Input: part model. Units: mm. Frame: model coordinates. A direction names the side the tool comes from. Round coordinates to 2 decimals unless told otherwise and drop trailing zeros. Order: outer loops, then holes, each group sorted by start corner. A loop starts at its lowest first (then second) coordinate and runs counter-clockwise, first axis right, second up.
Item 1: Cut plane D-D on y = 5.5. Give the number of separate pieces and of enclosed holes in the cut face, then the cut area to 3 significant figures.
Item 2: Cut plane C-C on x = 19. Output: boundary loops of the cut face in (y, z), then the cut area to 3 significant figures.
Item 3: Line query: L1, parallel to X at y = 1.5, z = 34; L2, parallel to Z at x = 0, y = 4.6; L3, parallel to X at y = 6.1, z = 0. Output: solid intervals per line, ascending.
Item 4: Cut plane A-A on z = 0. Output: boundary loops of the cut face in (x, y).
Item 5: First-contact query: pin 1 (4 mm diameter, centred on y = 3.5, z = 2, fed in from -X); pin 2 (0.8 mm diameter, centred on y = 6.5, z = 3, fed in from +X); pin 3 (2 mm diameter, centred on x = -37.5, y = 3.5, fed in from -Z). Flat tips, straight axial feed; report the tip coordinate or a pass-through.
Item 6: Reachability of faces 1 (the flat face through (25, 6, -4.5)), 2 (the flat face through (-16.61, 3.7, -23.68)), 3 (the flat face through (31, 6, 3.651)) from +Z, -Z, +X, -X, +Y, -Y: full face, straight path, thin tool, end or side. Return the list, or none.
Item 7: Cut plane B-B on x = 0. Output: boundary loops of the cut face in (y, z), then the cut area to 3 significant figures.
Item 8: Mould query, pull axis X, two halves, no side actions, for faces 4 (the flat face through (41.449, 4, 31)), 5 (the cylindrical face through (38.9, 3.8, 31.54)), 6 (the flat face through (36.559, 3.698, 36.648)), 7 (the flat face through (0, 0, -12)). Classes: released by +X, released by -X, zero draft, split by the parting line, or undercut.
```python
from build123d import *

# Parameters (mm, degrees)
SKETCH1_R           = 2.5
BOSS_EXTRUDE1_DEPTH = 7.5
FILLET3_R           = 1.5
SKETCH3_W           = 25.4
SKETCH3_H           = 9
CUT_EXTRUDE1_DEPTH  = 2
SKETCH2_W           = 24.748800006
SKETCH2_H           = 9
SKETCH2_W_2         = 9
SKETCH2_H_2         = 1.651
BOSS_EXTRUDE3_DEPTH = 3
SKETCH4_W           = 24.748800006
SKETCH4_H           = 9
BOSS_EXTRUDE4_DEPTH = 1


with BuildPart() as part:
    # Sketch1 → Boss-Extrude1 (new body)
    with BuildSketch(Plane(origin=(0, 0, 0), x_dir=(1, 0, 0), z_dir=(0, 1, 0))):
        Polygon((-41.448800006, 34.091704203), (-34.091704203, 41.448800006), (-27.292890359, 41.448800006), (-27.292890359, 34.363958171), (-5.628932188, 12.7), (5.628932188, 12.7), (27.292890359, 34.363958171), (27.292890359, 41.448800006), (34.091704203, 41.448800006), (41.448800006, 34.091704203), (41.448800006, 27.292890359), (34.363958171, 27.292890359), (12.7, 5.628932188), (12.7, -5.628932188), (34.363958171, -27.292890359), (41.448800006, -27.292890359), (41.448800006, -34.091704203), (34.091704203, -41.448800006), (27.292890359, -41.448800006), (27.292890359, -34.363958171), (5.628932188, -12.7), (-5.628932188, -12.7), (-27.292890359, -34.363958171), (-27.292890359, -41.448800006), (-34.091704203, -41.448800006), (-41.448800006, -34.091704203), (-41.448800006, -27.292890359), (-34.363958171, -27.292890359), (-12.7, -5.628932188), (-12.7, 5.628932188), (-34.363958171, 27.292890359), (-41.448800006, 27.292890359), align=None)
        with Locations(Location((0, 0, 0), (0, 0, 270))):
            Circle(SKETCH1_R, mode=Mode.SUBTRACT)
        Polygon((-39.798800006, 33.408251825), (-33.408251825, 39.798800006), (-29.292890359, 39.798800006), (-39.798800006, 29.292890359), align=None, mode=Mode.SUBTRACT)
        Polygon((-33.408251825, -39.798800006), (-29.292890359, -39.798800006), (-39.798800006, -29.292890359), (-39.798800006, -33.408251825), align=None, mode=Mode.SUBTRACT)
        Polygon((39.798800006, -33.408251825), (39.798800006, -29.292890359), (29.292890359, -39.798800006), (33.408251825, -39.798800006), align=None, mode=Mode.SUBTRACT)
        Polygon((33.408251825, 39.798800006), (39.798800006, 33.408251825), (39.798800006, 29.292890359), (29.292890359, 39.798800006), align=None, mode=Mode.SUBTRACT)
    extrude(amount=BOSS_EXTRUDE1_DEPTH)

    # Fillet3
    fillet3_edges = [part.edges().sort_by_distance(p)[0] for p in [
        (39.798800006, 3.75, 29.292890359),
        (29.292890359, 3.75, 39.798800006),
        (-29.292890359, 3.75, 39.798800006),
        (-39.798800006, 3.75, 29.292890359),
        (-39.798800006, 3.75, -29.292890359),
        (-29.292890359, 3.75, -39.798800006),
        (29.292890359, 3.75, -39.798800006),
        (39.798800006, 3.75, -29.292890359),
    ]]
    fillet(fillet3_edges, radius=FILLET3_R)

    # Sketch3 → Cut-Extrude1 (cut)
    with BuildSketch(Plane.XZ):
        Rectangle(SKETCH3_W, SKETCH3_H)
    extrude(amount=-CUT_EXTRUDE1_DEPTH, mode=Mode.SUBTRACT)

    # Sketch2 → Boss-Extrude3 (add)
    # profile 1 of 2: a face of its own
    with BuildSketch(Plane(origin=(0, 7.5, 0), x_dir=(1, 0, 0), z_dir=(0, 1, 0))):
        with Locations((25.074400003, 0)):
            Rectangle(SKETCH2_W, SKETCH2_H)
        with Locations((31.448800006, 2.8255)):
            Rectangle(SKETCH2_W_2, SKETCH2_H_2, mode=Mode.SUBTRACT)
        with Locations((31.448800006, -2.8255)):
            Rectangle(SKETCH2_W_2, SKETCH2_H_2, mode=Mode.SUBTRACT)
    # profile 2 of 2: a face of its own
    with BuildSketch(Plane(origin=(0, 7.5, 0), x_dir=(1, 0, 0), z_dir=(0, 1, 0))):
        with Locations((-25.074400003, 0)):
            Rectangle(SKETCH2_W, SKETCH2_H)
        with Locations((-31.448800006, 2.8255)):
            Rectangle(SKETCH2_W_2, SKETCH2_H_2, mode=Mode.SUBTRACT)
        with Locations((-31.448800006, -2.8255)):
            Rectangle(SKETCH2_W_2, SKETCH2_H_2, mode=Mode.SUBTRACT)
    extrude(amount=-BOSS_EXTRUDE3_DEPTH)

    # Sketch4 → Boss-Extrude4 (add)
    with BuildSketch(Plane.XZ.offset(-4.5)):
        with Locations((25.074400003, 0)):
            Rectangle(SKETCH4_W, SKETCH4_H)
        with Locations((-25.074400003, 0)):
            Rectangle(SKETCH4_W, SKETCH4_H)
    extrude(amount=BOSS_EXTRUDE4_DEPTH)


solid = part.part
```
From the geometry:
1. separate pieces: 1
1. enclosed holes: 9
1. area: 2,610 mm2
2. outline: (0, -26.07) - (7.5, -26.07) - (7.5, -11.93) - (0, -11.93) - close; (0, 11.93) - (7.5, 11.93) - (7.5, 26.07) - (0, 26.07) - close; (3.5, -4.5) - (7.5, -4.5) - (7.5, 4.5) - (3.5, 4.5) - close
2. area: 248 mm2
3. L1: x = -41.45 to -39.21, -35.09 to -26.93, 26.93 to 35.09, 39.21 to 41.45
3. L2: z = -12.7 to -2.5, 2.5 to 12.7
3. L3: x = -37.45 to -2.5, 2.5 to 37.45
4. outline: (-37.45, 3.5) - (-12.7, 3.5) - (-12.7, 2) - (-2.5, 2) - (-2.5, 7.5) - (-37.45, 7.5) - close; (2.5, 2) - (12.7, 2) - (12.7, 3.5) - (37.45, 3.5) - (37.45, 7.5) - (2.5, 7.5) - close
5. pin 1: stops at x = -37.45
5. pin 2: stops at x = 37.45
5. pin 3: stops at z = -39.04
6. face 1: +X, +Y, -Y
6. face 2: -Z, +Y, -Y
6. face 3: +Y
7. outline: (0, -12.7) - (7.5, -12.7) - (7.5, -2.5) - (2, -2.5) - (2, -4.5) - (0, -4.5) - close; (0, 4.5) - (2, 4.5) - (2, 2.5) - (7.5, 2.5) - (7.5, 12.7) - (0, 12.7) - close
7. area: 145 mm2
8. face 4: released by +X
8. face 5: undercut
8. face 6: undercut
8. face 7: zero draft
